Part print with two shaded views. Sizes in mm from the minimum x, y, z corner. A direction names the side the tool comes from. Round coordinates to 2 decimals unless told otherwise and drop trailing zeros. Write each loop counter-clockwise with the first axis right and the second up, starting at its lowest first coordinate (ties: lowest second). Pieces come first, ordered by that corner, then holes.
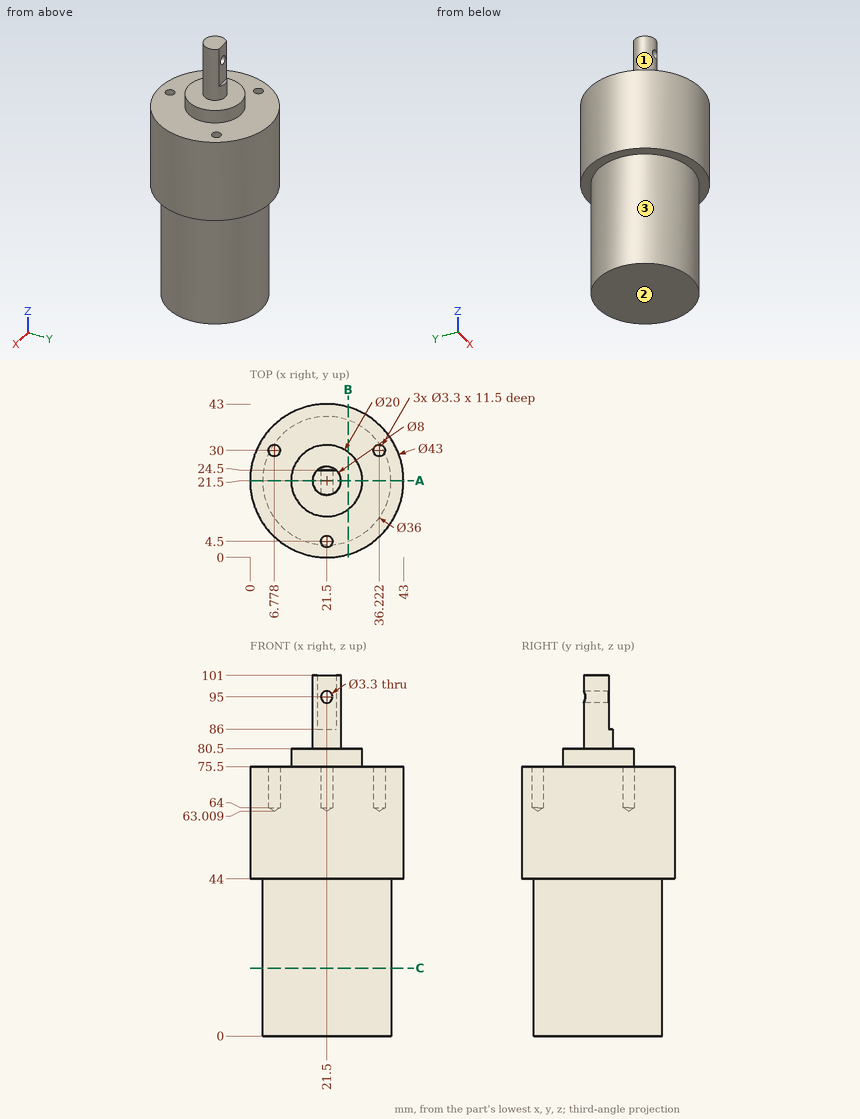
Q1. Which spindle directions (+Z, -Z, +X, -X, +Y, -Y) get a long thin tool onto all of the face, cutting with end or side? Do the marked faces 1, 2 and 3. Say none if no direction does.
Values follow:
face 1: +Z
face 2: -Z, +X, -X, +Y, -Y
face 3: -Z
Q2. Cut at B-B on x = 27.5. Write the cut outline in (y, z) (1 decimal).
Values follow:
outline: (0.9, 44) - (4.5, 44) - (4.5, 0) - (38.5, 0) - (38.5, 44) - (42.1, 44) - (42.1, 75.5) - (29.5, 75.5) - (29.5, 80.5) - (13.5, 80.5) - (13.5, 75.5) - (0.9, 75.5) - close
Q3. Cut at A-A on y = 21.5. Write the cut outline in (x, z), plus the area to 3 significant figures.
Values follow:
outline: (0, 44) - (3.5, 44) - (3.5, 0) - (39.5, 0) - (39.5, 44) - (43, 44) - (43, 75.5) - (31.5, 75.5) - (31.5, 80.5) - (25.5, 80.5) - (25.5, 101) - (17.5, 101) - (17.5, 80.5) - (11.5, 80.5) - (11.5, 75.5) - (0, 75.5) - close; hole circle Ø3.3 at (21.5, 95)
area: 3,190 mm2
Q4. Cut at C-C on z = 19. Write the cut outline in (x, y).
Values follow:
outline: circle Ø36 at (21.5, 21.5)
Q5. Wall check: L1, parallel to X at y = 30, z = 71; L2, parallel to Y at x = 18.5, z = 90.5 (1 decimal); L3, parallel to X at y = 20, z = 95. Give the ranges that are in metal, low to high.
Values follow:
L1: x = 1.75 to 5.13, 8.43 to 34.57, 37.87 to 41.25
L2: y = 18.9 to 24.1
L3: x = 17.79 to 19.85, 23.15 to 25.21
Q6. Drop flat-ended pins along their axis: pin 1 (2 mm diameter, centred on x = 36.22, y = 30, fed in from +Z); pin 2 (4 mm diameter, centred on x = 21, z = 77, fed in from -Y); pin 3 (1 mm diameter, centred on y = 20.5, z = 51.5, fed in from -X). Give the stop position or say it passes through.
Values follow:
pin 1: stops at z = 63.61
pin 2: stops at y = 0
pin 3: stops at x = 0.01
